Design review of the part built by this model. Coordinates are the model's own, in mm. A direction names the side the tool comes from. Give positions to 0.01 mm unless a question says otherwise; leave off trailing zeros. Loops run counter-clockwise (first coordinate to the right, second up) from the corner with the lowest first, then second, coordinate; pieces in that order, holes last. Notation, with made-up numbers: (73, 40) -> (108, 40) arc R11 ccw to (108, 45) -> close; hole circle Ø5 at (35.5, 23). An arc over 180 degrees is marked (long way). Answer in a Markdown table with one row per item. Add a question column.
(1) Consider section B-B on x = 2.5. Write out the cut boundary in (y, z).
(2) For pin 1 (6 mm diameter, centred on x = 17, z = -0.5, fed in from -Y); pin 2 (2 mm diameter, centred on x = 2.5, y = -1, fed in from -Z), all flat-tipped, find the tip position at first contact; note any pin that passes through.
(3) Consider section A-A on y = 0. Write out the cut boundary in (x, z), then the cut area to 3 significant figures.
(4) Consider section C-C on y = 3.5. Write out the cut boundary in (x, z).
(5) For line 1 (X direction, y = 5, z = -1.25); line 2 (Y direction, x = 18.75, z = 1.5); line 3 (Z direction, x = 18.5, y = 0.25), list the stretches that pass through material, from the lowest coordinate up.
(6) For faces 1 (the flat face through (0, 0.1, -3.4)), 2 (the flat face through (-3, 0, 0)), list the 3-axis set-ups (+Z, -Z, +X, -X, +Y, -Y) from which the entire face can be reached by the end or side of a thin tool; tool diameter is ignored.
Autodesk Inventor part; units mm, degrees
ref_plane "Work Plane1" through (1.525, 0, 0) normal (0, 0, 1) x (1, 0, 0)
ref_plane "YZ Plane" through (0, 0, 0) normal (1, 0, 0) x (0, 1, 0)
ref_plane "XZ Plane" through (0, 0, 0) normal (0, 1, 0) x (-1, 0, 0)
sketch "Sketch1" plane through (0, 0, 0) normal (0, 0, 1) x (1, 0, 0)
  line L0 (0, 3) -> (20, 3)
  line L1 (20, 3) -> (20, 0)
  line L2 (20, 0) -> (0, 0)
  line L3 (-4, 0) -> (24, 0)
  line L4 (0, -0.6) -> (0, 3.6)
  line L5 (0, 3) -> (0, 0)
  dimension "d2" = 6
  dimension "d59" = 20
revolve "Body" add sketch "Sketch1" angle 360 about axis through (20, 0, 0) along (-1, 0, 0)
sketch "Sketch2" plane through (0, 0, 0) normal (-1, 0, 0) x (0, 0, 1)
  line L0 (0, 5.7735) -> (5, 2.8868)
  line L1 (5, 2.8868) -> (5, -2.8868)
  line L2 (5, -2.8868) -> (0, -5.7735)
  line L3 (0, -5.7735) -> (-5, -2.8868)
  line L4 (-5, -2.8868) -> (-5, 2.8868)
  line L5 (-5, 2.8868) -> (0, 5.7735)
  line L6 (-7, 0) -> (7, 0)
  line L7 (0, 8.0829) -> (0, -8.0829)
  point P0 (0, 0)
  point P1 (0, 0)
  dimension "d11" = 10
extrude "Head" add sketch "Sketch2" along normal blind 4
sketch "Sketch4" plane through (0, 0, 0) normal (0, 0, 1) x (1, 0, 0)
  line L0 (-3.4226, 6) -> (-4, 5)
  line L1 (-1.1, 0) -> (-0.234, 0)
  line L2 (-4.7532, 0) -> (0.5192, 0)
  line L3 (-4, 6) -> (-3.4226, 6)
  line L4 (-4, 5) -> (-4, 6)
  line L5 (0, 7.2) -> (0, -1.2)
  dimension "d65" = 10
  dimension "d67" = 30
  dimension "d68" = 12
  dimension "d69" = 4
revolve "Chamfer1" cut sketch "Sketch4" angle 360 about axis through (-1.1, 0, 0) along (1, 0, 0)
thread "Thread"
chamfer "Chamfer2" distance 0.6135 distance2 0.6136 1 edges at (20, -3, 0) measured on face at (20, -0.301, 1.1526)
fillet "Fillet2" radius 0.25 1 edges at (0, -3, 0)
ref_plane "Work Plane1" through (1.525, 0, 0) normal (0, 0, 1) x (1, 0, 0)
sketch "Sketch7" plane through (-4, 0, 0) normal (-1, 0, 0) x (0, 0, 1)
  arc A0 (2.5, 4.3301) -> (-2.5, 4.3301) centre (0, 0) ccw
  circle A1 centre (0, 0) radius 6.6144
extrude "Extrusion5" cut sketch "Sketch7" against normal blind 1
equation "\"d2\" = GD"
equation "\"d59\" = NLG"
equation "\"d11\" = SW"
equation "\"d3\" = KOH"
equation "\"d71\" = RR"
equation "\"d15\" = GEL"
equation "\"d6\" = -0.5 * SPD + 0.5 * GD"
equation "\"d65\" = SW"
equation "\"d67\" = ANG1"
equation "\"d68\" = 1.2 * SW"
equation "\"d69\" = KOH"
equation "\"NLG\" = 20"
equation "\"GD\" = NND"
equation "\"BDM\" = NND"
equation "\"KOH\" = 4"
equation "\"GEL\" = 19"
equation "\"SW\" = 10"
equation "\"SPD\" = NND - 1.2269 * PTC"
equation "\"SD2\" = NND"
equation "\"SD\" = 0"
equation "\"ANG1\" = 30deg"
equation "\"GAL\" = 0.61345 * PTC"
equation "\"GUL\" = 0.61345 * PTC"
equation "\"RR\" = 0.25"
equation "\"RR1\" = 0.1"
equation "\"WFT\" = 0"
equation "\"GD1\" = THREADDIA - 1.2269 * PTC"
equation "\"THREADDIA\" = 6"
equation "\"TOA\" = 30deg"
equation "\"FAWI\" = 90deg"
equation "\"PTC\" = 1"
equation "\"NND\" = 6"
equation "\"E0\" = 1.155 * SW"
properties part number "Hexagon bolt GB/T 5781 M6 x 20" material "Steel, Mild"
Values follow:
| question | item | result |
|---|---|---|
| 1 | outline | circle Ø6 at (0, 0) |
| 2 | pin 1 | y = -3 |
| 2 | pin 2 | z = -3 |
| 3 | outline | (-3, -5) -> (0, -5) -> (0, -3.25) arc R0.25 cw to (0.25, -3) -> (19.39, -3) -> (20, -2.39) -> (20, 2.39) -> (19.39, 3) -> (0.25, 3) arc R0.25 cw to (0, 3.25) -> (0, 5) -> (-3, 5) -> close |
| 3 | area | 150 mm2 |
| 4 | outline | (-3, -3.94) -> (0, -3.94) -> (0, 3.94) -> (-3, 3.94) -> close |
| 5 | line 1 | -3 to 0 |
| 5 | line 2 | -2.6 to 2.6 |
| 5 | line 3 | -2.99 to 2.99 |
| 6 | face 1 | +X |
| 6 | face 2 | +Z, -Z, -X, +Y, -Y |
